from build123d import *

# Parameters (mm, degrees)
BOSS_EXTRUDE1_DEPTH = 31
CUT_EXTRUDE1_REACH  = 97.635
SKETCH2_R           = 1.25
CUT_EXTRUDE2_REACH  = 90.781
SKETCH3_W           = 37.5
SKETCH3_H           = 16
CUT_EXTRUDE3_REACH  = 90.781
SKETCH4_R           = 1.25
CUT_EXTRUDE4_REACH  = 90.781
SKETCH6_W           = 36
SKETCH6_H           = 15
CUT_EXTRUDE5_REACH  = 90.781
FILLET1_R           = 5


with BuildPart() as part:
    # Sketch1 → Boss-Extrude1 (new, symmetric)
    with BuildSketch(Plane.XY):
        Polygon((-36, 0), (0, 0), (0, -75), (8, -75), (8, 8), (-36, 8), align=None)
    extrude(amount=BOSS_EXTRUDE1_DEPTH, both=True)

    # Sketch2 → Cut-Extrude1 (cut, up to next)
    with BuildSketch(Plane(origin=(0, 8, 0), x_dir=(1, 0, 0), z_dir=(0, 1, 0)), mode=Mode.PRIVATE) as cut_extrude1_sk1:
        with Locations(Location((-32.070312755, -12.070312755, 0), (0, 0, 180))):
            Circle(SKETCH2_R)
    cut_extrude1_tool1 = extrude(cut_extrude1_sk1.sketch, amount=-CUT_EXTRUDE1_REACH, mode=Mode.PRIVATE) & part.part
    # Sketch2 → Cut-Extrude1 (cut, up to next)
    with BuildSketch(Plane(origin=(0, 8, 0), x_dir=(1, 0, 0), z_dir=(0, 1, 0)), mode=Mode.PRIVATE) as cut_extrude1_sk2:
        with Locations(Location((-32.070312755, 12.070312755, 0), (0, 0, 180))):
            Circle(SKETCH2_R)
    cut_extrude1_tool2 = extrude(cut_extrude1_sk2.sketch, amount=-CUT_EXTRUDE1_REACH, mode=Mode.PRIVATE) & part.part
    # Sketch2 → Cut-Extrude1 (cut, up to next)
    with BuildSketch(Plane(origin=(0, 8, 0), x_dir=(1, 0, 0), z_dir=(0, 1, 0)), mode=Mode.PRIVATE) as cut_extrude1_sk3:
        with Locations(Location((-7.929687245, 12.070312755, 0), (0, 0, 180))):
            Circle(SKETCH2_R)
    cut_extrude1_tool3 = extrude(cut_extrude1_sk3.sketch, amount=-CUT_EXTRUDE1_REACH, mode=Mode.PRIVATE) & part.part
    # Sketch2 → Cut-Extrude1 (cut, up to next)
    with BuildSketch(Plane(origin=(0, 8, 0), x_dir=(1, 0, 0), z_dir=(0, 1, 0)), mode=Mode.PRIVATE) as cut_extrude1_sk4:
        with Locations(Location((-7.929687245, -12.070312755, 0), (0, 0, 180))):
            Circle(SKETCH2_R)
    cut_extrude1_tool4 = extrude(cut_extrude1_sk4.sketch, amount=-CUT_EXTRUDE1_REACH, mode=Mode.PRIVATE) & part.part
    # Sketch2 → Cut-Extrude1 (cut, up to next)
    with BuildSketch(Plane(origin=(0, 8, 0), x_dir=(1, 0, 0), z_dir=(0, 1, 0)), mode=Mode.PRIVATE) as cut_extrude1_sk5:
        Polygon((-13, 4.041451884), (-20, 8.082903769), (-27, 4.041451884), (-27, -4.041451884), (-20, -8.082903769), (-13, -4.041451884), align=None)
    cut_extrude1_tool5 = extrude(cut_extrude1_sk5.sketch, amount=-CUT_EXTRUDE1_REACH, mode=Mode.PRIVATE) & part.part
    add(cut_extrude1_tool1.solids().sort_by_distance((-32.070313, 8, 12.070313))[0], mode=Mode.SUBTRACT)
    add(cut_extrude1_tool2.solids().sort_by_distance((-32.070313, 8, -12.070313))[0], mode=Mode.SUBTRACT)
    add(cut_extrude1_tool3.solids().sort_by_distance((-7.929687, 8, -12.070313))[0], mode=Mode.SUBTRACT)
    add(cut_extrude1_tool4.solids().sort_by_distance((-7.929687, 8, 12.070313))[0], mode=Mode.SUBTRACT)
    add(cut_extrude1_tool5.solids().sort_by_distance((-20, 8, 0))[0], mode=Mode.SUBTRACT)

    # Sketch3 → Cut-Extrude2 (cut, up to next)
    with BuildSketch(Plane.ZY, mode=Mode.PRIVATE) as cut_extrude2_sk1:
        with Locations((-6.81, -67)):
            Rectangle(SKETCH3_W, SKETCH3_H)
    cut_extrude2_tool1 = extrude(cut_extrude2_sk1.sketch, amount=-CUT_EXTRUDE2_REACH, mode=Mode.PRIVATE) & part.part
    add(cut_extrude2_tool1.solids().sort_by_distance((0, -67, -6.81))[0], mode=Mode.SUBTRACT)

    # Sketch4 → Cut-Extrude3 (cut, up to next)
    with BuildSketch(Plane.ZY, mode=Mode.PRIVATE) as cut_extrude3_sk1:
        with Locations(Location((14.29, -70.6, 0), (0, 0, 270))):
            Circle(SKETCH4_R)
    cut_extrude3_tool1 = extrude(cut_extrude3_sk1.sketch, amount=-CUT_EXTRUDE3_REACH, mode=Mode.PRIVATE) & part.part
    # Sketch4 → Cut-Extrude3 (cut, up to next)
    with BuildSketch(Plane.ZY, mode=Mode.PRIVATE) as cut_extrude3_sk2:
        with Locations(Location((14.29, -63.4, 0), (0, 0, 270))):
            Circle(SKETCH4_R)
    cut_extrude3_tool2 = extrude(cut_extrude3_sk2.sketch, amount=-CUT_EXTRUDE3_REACH, mode=Mode.PRIVATE) & part.part
    # Sketch4 → Cut-Extrude3 (cut, up to next)
    with BuildSketch(Plane.ZY, mode=Mode.PRIVATE) as cut_extrude3_sk3:
        with Locations(Location((-27.91, -63.4, 0), (0, 0, 270))):
            Circle(SKETCH4_R)
    cut_extrude3_tool3 = extrude(cut_extrude3_sk3.sketch, amount=-CUT_EXTRUDE3_REACH, mode=Mode.PRIVATE) & part.part
    # Sketch4 → Cut-Extrude3 (cut, up to next)
    with BuildSketch(Plane.ZY, mode=Mode.PRIVATE) as cut_extrude3_sk4:
        with Locations(Location((-27.91, -70.6, 0), (0, 0, 270))):
            Circle(SKETCH4_R)
    cut_extrude3_tool4 = extrude(cut_extrude3_sk4.sketch, amount=-CUT_EXTRUDE3_REACH, mode=Mode.PRIVATE) & part.part
    add(cut_extrude3_tool1.solids().sort_by_distance((0, -70.6, 14.29))[0], mode=Mode.SUBTRACT)
    add(cut_extrude3_tool2.solids().sort_by_distance((0, -63.4, 14.29))[0], mode=Mode.SUBTRACT)
    add(cut_extrude3_tool3.solids().sort_by_distance((0, -63.4, -27.91))[0], mode=Mode.SUBTRACT)
    add(cut_extrude3_tool4.solids().sort_by_distance((0, -70.6, -27.91))[0], mode=Mode.SUBTRACT)

    # Sketch6 → Cut-Extrude4 (cut, up to next)
    with BuildSketch(Plane.XZ, mode=Mode.PRIVATE) as cut_extrude4_sk1:
        with Locations((-18, -23.5)):
            Rectangle(SKETCH6_W, SKETCH6_H)
    cut_extrude4_tool1 = extrude(cut_extrude4_sk1.sketch, amount=-CUT_EXTRUDE4_REACH, mode=Mode.PRIVATE) & part.part
    # Sketch6 → Cut-Extrude4 (cut, up to next)
    with BuildSketch(Plane.XZ, mode=Mode.PRIVATE) as cut_extrude4_sk2:
        with Locations((-18, 23.5)):
            Rectangle(SKETCH6_W, SKETCH6_H)
    cut_extrude4_tool2 = extrude(cut_extrude4_sk2.sketch, amount=-CUT_EXTRUDE4_REACH, mode=Mode.PRIVATE) & part.part
    add(cut_extrude4_tool1.solids().sort_by_distance((-18, 0, -23.5))[0], mode=Mode.SUBTRACT)
    add(cut_extrude4_tool2.solids().sort_by_distance((-18, 0, 23.5))[0], mode=Mode.SUBTRACT)

    # Sketch7 → Cut-Extrude5 (cut, up to next)
    with BuildSketch(Plane.ZY, mode=Mode.PRIVATE) as cut_extrude5_sk1:
        Polygon((-16, 0), (-31, -26), (-31, 8), (-16, 8), align=None)
    cut_extrude5_tool1 = extrude(cut_extrude5_sk1.sketch, amount=-CUT_EXTRUDE5_REACH, mode=Mode.PRIVATE) & part.part
    # Sketch7 → Cut-Extrude5 (cut, up to next)
    with BuildSketch(Plane.ZY, mode=Mode.PRIVATE) as cut_extrude5_sk2:
        Polygon((16, 0), (21, -26), (21, -75), (31, -75), (31, 8), (16, 8), align=None)
    cut_extrude5_tool2 = extrude(cut_extrude5_sk2.sketch, amount=-CUT_EXTRUDE5_REACH, mode=Mode.PRIVATE) & part.part
    add(cut_extrude5_tool1.solids().sort_by_distance((0, -3.84127, -25.047619))[0], mode=Mode.SUBTRACT)
    add(cut_extrude5_tool2.solids().sort_by_distance((0, -30.16934, 25.215686))[0], mode=Mode.SUBTRACT)

    # Fillet1
    fillet1_edges = [part.edges().sort_by_distance(p)[0] for p in [
        (0, 0, 0),
    ]]
    fillet(fillet1_edges, radius=FILLET1_R)


solid = part.part
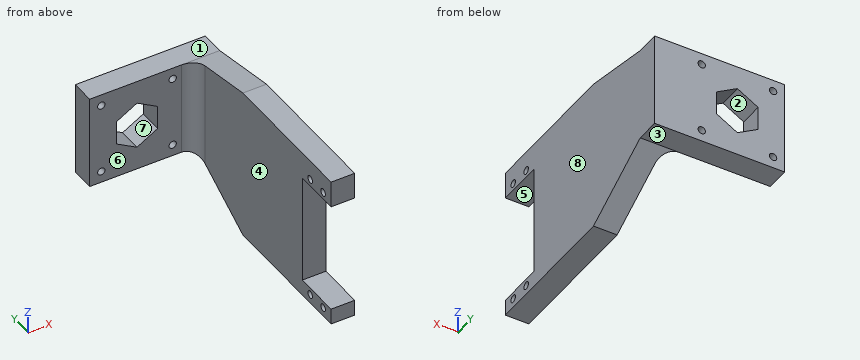
Geometry: final body of the model. Coordinates: model frame, mm. Face numbers are marked on the shaded views. A direction names the side the tool comes from. Give positions to 0.01 mm unless a question says otherwise; leave off trailing zeros. Write each loop counter-clockwise with the first axis right and the second up, starting at its lowest first coordinate (ties: lowest second). Pieces come first, ordered by that corner, then holes.
(1) First-contact query: P1, Ø4, axis at x = -24.5, y = 5.5, coming from the -Z side; P2, Ø2.5, axis at x = -21, y = 3.5, coming from the +Z side; P3, Ø15.5, axis at x = -27, z = -2.5, coming from the -Y side; P4, Ø2, axis at x = -32.07, z = 12.07, coming from the +Y side. Flat tips, straight axial feed; report the tip coordinate or a pass-through.
(2) Ray query, line 1 (Z direction, x = 2.25, y = -70.6); line 2 (Z direction, x = 4, y = -70); line 3 (X direction, y = -44.5, z = 13.5). Return the intervals inside material, ascending.
(3) Cut plane A-A, the plane z = 0.5. Return loops of the section in (x, y).
(4) Mould query, pull axis X, two halves, no side actions, for the marked faces 6, 7 and 8. Classes: released by +X, released by -X, zero draft, split by the parting line, or undercut.
(5) Cut plane B-B, the plane y = -63.4. Return loops of the section in (x, z).
(6) Cut plane D-D, the plane x = -21.5. Return loops of the section in (y, z).
(7) Access query for the marked faces 1, 2, 3, 4 and 5. Directions: +Z, -Z, +X, -X, +Y, -Y. A direction counts if a zero-diameter tool reaches every point of the face in a straight line with its end or side. Return the directions, or none.
(8) Cut plane C-C, the plane z = 14.29. Return loops of the section in (x, y).
Values follow:
1. P1: stops at z = -16
1. P2: stops at z = 16
1. P3: stops at y = 0
1. P4: passes through
2. line 1: z = -31 to -29.16, -26.66 to -25.56, 11.94 to 13.04, 15.54 to 21
2. line 2: z = -31 to -29.01, -26.81 to -25.56, 11.94 to 13.19, 15.39 to 21
2. line 3: x = 0 to 8
3. outline: (-36, 0) - (-27, 0) - (-27, 8) - (-36, 8) - close; (-13, 0) - (-5, 0) arc R5 cw to (0, -5) - (0, -59) - (8, -59) - (8, 8) - (-13, 8) - close
4. face 6: zero draft
4. face 7: undercut
4. face 8: released by +X
5. outline: (0, -31) - (8, -31) - (8, -29.16) - (0, -29.16) - close; (0, -26.66) - (8, -26.66) - (8, -25.56) - (0, -25.56) - close; (0, 11.94) - (8, 11.94) - (8, 13.04) - (0, 13.04) - close; (0, 15.54) - (8, 15.54) - (8, 21) - (0, 21) - close
6. outline: (0, -16) - (8, -16) - (8, -7.22) - (0, -7.22) - close; (0, 7.22) - (8, 7.22) - (8, 16) - (0, 16) - close
7. face 1: +Z, +X, -X, +Y
7. face 2: +Y, -Y
7. face 3: -Z, +X, -X, +Y
7. face 4: +Z, -Z, -X, -Y
7. face 5: +X, -X, -Y
8. outline: (-36, 0) - (-5, 0) arc R5 cw to (0, -5) - (0, -62.15) - (8, -62.15) - (8, 8) - (-36, 8) - close; (0, -75) - (8, -75) - (8, -71.85) - (0, -71.85) - close; (0, -69.35) - (8, -69.35) - (8, -64.65) - (0, -64.65) - close
